The listing builds one solid part. Answer for the finished solid, in the listing's coordinates (mm). Face numbers are marked on the shaded views. Round coordinates to 2 decimals unless told otherwise and drop trailing zeros. Loops run counter-clockwise (first coordinate to the right, second up) from the corner with the lowest first, then second, coordinate; pieces in that order, holes last. Notation, with made-up numbers: M -20,80.25 L 3,80.25 A14 ccw 3,92.25 Z; hole C 88,14 d5. An arc over 180 degrees is marked long. Put each result on its own line as item: value. Start each with the question number.
(1) Section B-B, the plane x = 2 is taken. Determine the outline of the cut face in (y, z).
(2) Determine the mould class of the marked faces 1, 2, 3 and 4 for opening direction Z: released by +Z, released by -Z, zero draft, split by the parting line, or undercut.
(3) Section A-A, the plane z = -3 is taken. Determine the outline of the cut face in (x, y), then the cut area to 3 significant figures.
(4) Section D-D, the plane x = -5.5 is taken. Determine the outline of the cut face in (y, z), then the cut area to 3 significant figures.
(5) Section C-C, the plane y = 1 is taken. Determine the outline of the cut face in (x, z).
(6) Straight lines are drawn through the part: line 1 (Y direction, x = 7.5, z = 31); line 2 (Z direction, x = -2, y = 6.75); line 3 (Z direction, x = -3, y = 9.75). For each, find the intervals that lie inside material, in ascending order.
(7) Flat-ended cylindrical pins translate along their axes: P1, Ø7.5, axis at x = 2.5, z = 3.5, coming from the +Y side; P2, Ø1, axis at x = -9, y = 9, coming from the +Z side. Find the tip coordinate at first contact, or state that the pin passes through.
```python
from build123d import *

# Parameters (mm, degrees)
SKETCH1_W           = 45.01572081
SKETCH1_H           = 71
SKETCH1_R           = 1.75
SKETCH1_R_2         = 4.5
BOSS_EXTRUDE1_DEPTH = 5
SKETCH2_R           = 15.2
SKETCH2_R_2         = 12.2
BOSS_EXTRUDE2_DEPTH = 6
SKETCH3_R           = 1.5
CUT_EXTRUDE1_DEPTH  = 60
SKETCH4_R           = 12.2
SKETCH4_R_2         = 12.15
BOSS_EXTRUDE3_DEPTH = 6
SKETCH5_R           = 1.5
SKETCH5_R_2         = 1
SKETCH5_R_3         = 1.75
SKETCH5_R_4         = 1.25
BOSS_EXTRUDE4_DEPTH = 5


with BuildPart() as part:
    # Sketch1 → Boss-Extrude1 (new body)
    with BuildSketch(Plane(origin=(0, 0, 0), x_dir=(1, 0, 0), z_dir=(0, 1, 0))):
        with Locations((0.136395343, 0.409186029)):
            Rectangle(SKETCH1_W, SKETCH1_H)
        with Locations((17.636395343, -7.590813971)):
            Circle(SKETCH1_R, mode=Mode.SUBTRACT)
        with Locations((0.136395343, 0.409186029)):
            Circle(SKETCH1_R_2, mode=Mode.SUBTRACT)
        with Locations((-17.363604657, -7.590813971)):
            Circle(SKETCH1_R, mode=Mode.SUBTRACT)
    extrude(amount=BOSS_EXTRUDE1_DEPTH)

    # Sketch2 → Boss-Extrude2 (add)
    with BuildSketch(Plane(origin=(0, 5, 0), x_dir=(1, 0, 0), z_dir=(0, 1, 0))):
        with Locations((0.136395343, 0.409186029)):
            Circle(SKETCH2_R)
        with Locations((0.136395343, 0.409186029)):
            Circle(SKETCH2_R_2, mode=Mode.SUBTRACT)
    extrude(amount=BOSS_EXTRUDE2_DEPTH)

    # Sketch3 → Cut-Extrude1 (cut)
    with BuildSketch(Plane.XZ):
        with Locations((18.022935404, 29.969493628)):
            Circle(SKETCH3_R)
        with Locations((-17.750144718, 29.969493628)):
            Circle(SKETCH3_R)
        with Locations((-17.750144718, -30.787865685)):
            Circle(SKETCH3_R)
        with Locations((18.022935404, -30.787865685)):
            Circle(SKETCH3_R)
    extrude(amount=-CUT_EXTRUDE1_DEPTH, mode=Mode.SUBTRACT)

    # Sketch4 → Boss-Extrude3 (add)
    with BuildSketch(Plane(origin=(0, 11, 0), x_dir=(1, 0, 0), z_dir=(0, 1, 0))):
        with Locations((0.136395343, 0.409186029)):
            Circle(SKETCH4_R)
        with Locations((0.136395343, 0.409186029)):
            Circle(SKETCH4_R_2, mode=Mode.SUBTRACT)
    extrude(amount=-BOSS_EXTRUDE3_DEPTH)

    # Sketch5 → Boss-Extrude4 (add)
    with BuildSketch(Plane(origin=(0, 5, 0), x_dir=(1, 0, 0), z_dir=(0, 1, 0))):
        with Locations((-17.750144718, -29.969493628)):
            Circle(SKETCH5_R)
        with Locations((-17.750144718, -29.969493628)):
            Circle(SKETCH5_R_2, mode=Mode.SUBTRACT)
        with Locations((18.022935404, -29.969493628)):
            Circle(SKETCH5_R)
        with Locations((18.022935404, -29.969493628)):
            Circle(SKETCH5_R_2, mode=Mode.SUBTRACT)
        with Locations((17.636395343, -7.590813971)):
            Circle(SKETCH5_R_3)
        with Locations((17.636395343, -7.590813971)):
            Circle(SKETCH5_R_4, mode=Mode.SUBTRACT)
        with Locations((-17.363604657, -7.590813971)):
            Circle(SKETCH5_R_3)
        with Locations((-17.363604657, -7.590813971)):
            Circle(SKETCH5_R_4, mode=Mode.SUBTRACT)
        with Locations((-17.750144718, 30.787865685)):
            Circle(SKETCH5_R)
        with Locations((-17.750144718, 30.787865685)):
            Circle(SKETCH5_R_2, mode=Mode.SUBTRACT)
        with Locations((18.022935404, 30.787865685)):
            Circle(SKETCH5_R)
        with Locations((18.022935404, 30.787865685)):
            Circle(SKETCH5_R_2, mode=Mode.SUBTRACT)
    extrude(amount=-BOSS_EXTRUDE4_DEPTH)


solid = part.part
```
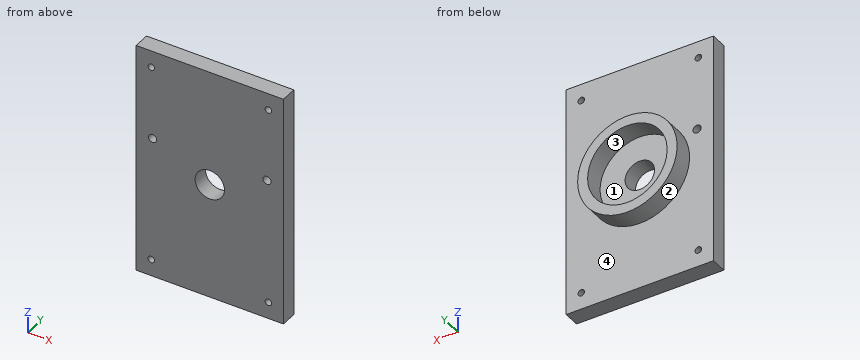
Recorded:
1. outline: M 0,-35.91 L 5,-35.91 L 5,-15.49 L 11,-15.49 L 11,-12.42 L 5,-12.42 L 5,-4.51 L 0,-4.51 Z; M 0,3.69 L 5,3.69 L 5,11.6 L 11,11.6 L 11,14.68 L 5,14.68 L 5,35.09 L 0,35.09 Z
2. face 1: undercut
2. face 2: split by the parting line
2. face 3: undercut
2. face 4: zero draft
3. outline: M -22.37,0 L -3.54,0 L -3.54,5 L -11.73,5 L -11.73,11 L -14.84,11 L -14.84,5 L -22.37,5 Z; M 3.82,0 L 22.64,0 L 22.64,5 L 15.11,5 L 15.11,11 L 12.01,11 L 12.01,5 L 3.82,5 Z
3. area: 226 mm²
4. outline: M 0,-35.91 L 5,-35.91 L 5,-14.53 L 11,-14.53 L 11,-11.17 L 5,-11.17 L 5,10.35 L 11,10.35 L 11,13.71 L 5,13.71 L 5,35.09 L 0,35.09 Z
4. area: 395 mm²
5. outline: M -22.37,-35.91 L 22.64,-35.91 L 22.64,35.09 L -22.37,35.09 Z; hole C -17.75,-30.79 d2; hole C -17.75,29.97 d2; hole C -17.36,7.59 d2.5; hole C 0.14,-0.41 d9; hole C 17.64,7.59 d2.5; hole C 18.02,-30.79 d2; hole C 18.02,29.97 d2
6. line 1: y = 0 to 5
6. line 2: z = -15.46 to -12.37, 11.55 to 14.64
6. line 3: z = -15.28 to -12.15, 11.33 to 14.46
7. P1: stops at y = 5
7. P2: stops at z = 12.1
